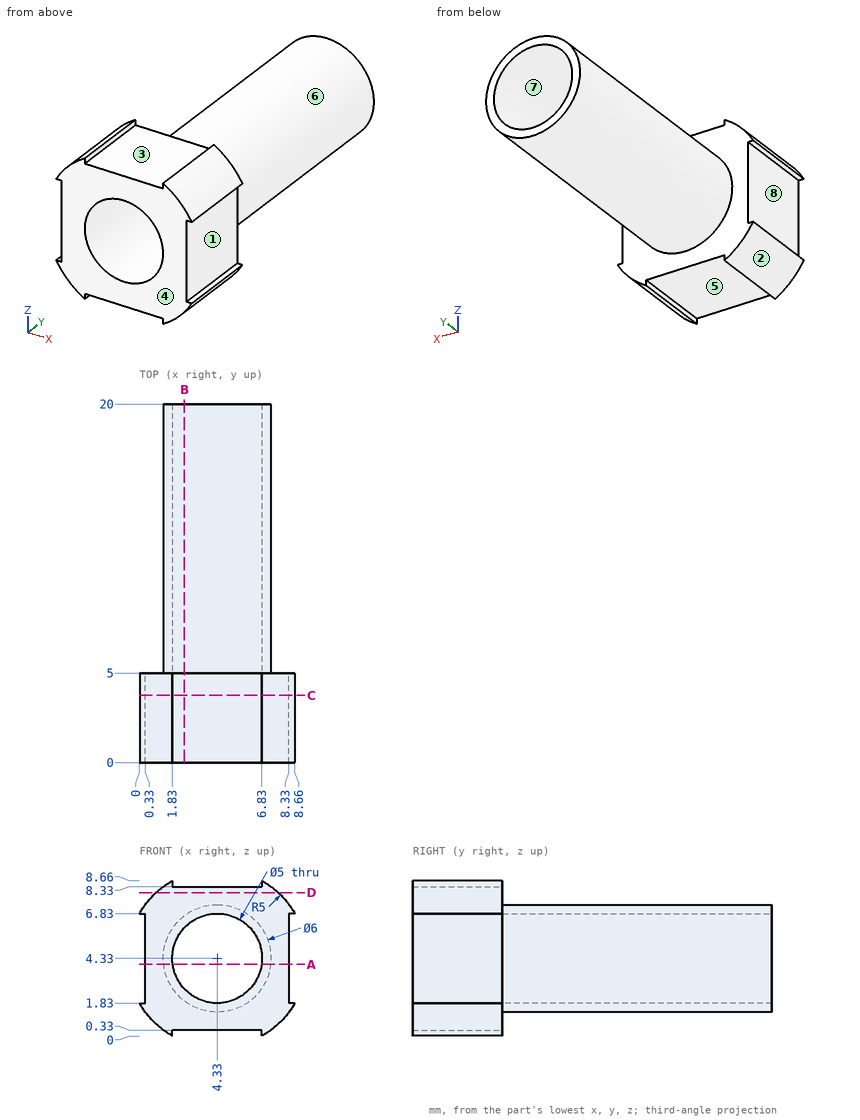
Print and shaded views of the part. All mm, measured from the part's lowest x, y and z. A direction names the side the tool comes from. Coordinates: 2 decimals unless noted, no trailing zeros. Loops run counter-clockwise (first coordinate to the right, second up) from the corner with the lowest first, then second, coordinate; pieces in that order, holes last. Notation, with made-up numbers: (10.5, 25) -> (66.5, 25) arc R11 ccw to (66.5, 46) -> close; hole circle Ø9 at (-16.5, 38.25). An arc over 180 degrees is marked (long way). Use one line per item in the form item = value. Start each with the question number.
(1) Cut at B-B on x = 2.5. Give the cut face in (y, z).
(2) Probe probe 1 along Z at (x, y) = (4.25, 2); probe 2 along Y at (x, z) = (0.5, 1.5). List the from-to ranges inside material, lowest first. Write a range as from..to.
(3) Cut at D-D on z = 8. Give the cut face in (x, y).
(4) Tool access for the marked faces 4, 5, 6, 7 and 8: list every direction of +Z, -Z, +X, -X, +Y, -Y with a clear straight run to the whole face (end or side of a thin tool).
(5) Pull direction Z, two halves, no side cores. Call the marked faces 1, 2 and 3: pulls with the +Z half, pulls with the -Z half, needs draft (parallel to the pull), parting line crosses it, or undercut.
(6) Cut at C-C on y = 3.75. Give the cut face in (x, z).
(7) Flat gauge pins, fed straight in: pin 1 (4 mm diameter, centred on y = 14, z = 1.5, fed in from -X); pin 2 (4 mm diameter, centred on x = 4.5, y = 11, fed in from +Z); pin 3 (1 mm diameter, centred on x = 5.5, y = 16.5, fed in from -Z); pin 4 (5 mm diameter, centred on x = 4, z = 4.5, fed in from +Y). Where does each tip first touch, or does it go through?
(8) Cut at A-A on z = 4. Give the cut face in (x, y).
Values:
q1.outline = (0, 0.33) -> (5, 0.33) -> (5, 1.95) -> (20, 1.95) -> (20, 2.63) -> (0, 2.63) -> close; (0, 6.03) -> (20, 6.03) -> (20, 6.71) -> (5, 6.71) -> (5, 8.33) -> (0, 8.33) -> close
q2.probe_1 = 0.33..1.83, 6.83..8.33
q2.probe_2 = 0..5
q3.outline = (0.93, 0) -> (7.73, 0) -> (7.73, 5) -> (0.93, 5) -> close
q4.face_4 = +Z, -Z, +X, -X, -Y
q4.face_5 = -Z, +Y, -Y
q4.face_6 = +Y
q4.face_7 = +Y, -Y
q4.face_8 = -X, +Y, -Y
q5.face_1 = undercut
q5.face_2 = pulls with the -Z half
q5.face_3 = pulls with the +Z half
q6.outline = (0, 1.83) arc R5 ccw to (1.83, 0) -> (1.83, 0.33) -> (6.83, 0.33) -> (6.83, 0) arc R5 ccw to (8.66, 1.83) -> (8.33, 1.83) -> (8.33, 6.83) -> (8.66, 6.83) arc R5 ccw to (6.83, 8.66) -> (6.83, 8.33) -> (1.83, 8.33) -> (1.83, 8.66) arc R5 ccw to (0, 6.83) -> (0.33, 6.83) -> (0.33, 1.83) -> close; hole circle Ø5 at (4.33, 4.33)
q7.pin_1 = 1.45
q7.pin_2 = 7.33
q7.pin_3 = 1.41
q7.pin_4 = 20
q8.outline = (0.33, 0) -> (1.85, 0) -> (1.85, 20) -> (1.35, 20) -> (1.35, 5) -> (0.33, 5) -> close; (6.81, 0) -> (8.33, 0) -> (8.33, 5) -> (7.31, 5) -> (7.31, 20) -> (6.81, 20) -> close
